Part model, mm, in its own coordinate system. Round coordinates to 2 decimals unless told otherwise and drop trailing zeros. Write each loop counter-clockwise with the first axis right and the second up, starting at its lowest first coordinate (ties: lowest second). Pieces come first, ordered by that corner, then holes. Notation, with made-up numbers: M 25,-24 L 48,-24 A9 ccw 48,-14 Z; hole C 15.25,46.5 d6. An arc over 180 degrees is marked long. Use one line per item in the form item = value. Start each with the question number.
Item 1: Flat gauge pins, fed straight in: pin 1 Ø3 at (y, z) = (3, 59) entering from +X; pin 2 Ø1.9 at (y, z) = (4.5, 45.5) entering from -X. Where does each tip first touch, or does it go through?
Item 2: Cut at A-A, the plane y = 4.5. State how many separate pieces and enclosed holes the cut face has, then the cut area to 3 significant figures.
Item 3: Probe L1, parallel to X at y = 2.5, z = 107; L2, parallel to X at y = 2.75, z = 9; L3, parallel to Z at x = 50.5, y = 3.25. List the from-to ranges inside material, lowest first.
Item 4: Cut at C-C, the plane x = 3. Give the cut face in (y, z), then the cut area to 3 significant figures.
Item 5: Cut at B-B, the plane z = 47. Give the cut face in (x, y).
Item 6: Cut at D-D, the plane z = 7. Give the cut face in (x, y).
from build123d import *

# Parameters (mm, degrees)
SKETCH1_R           = 2.6
SKETCH1_R_2         = 4
SKETCH1_R_3         = 6.35
SKETCH1_R_4         = 1
BOSS_EXTRUDE2_DEPTH = 6.3


with BuildPart() as part:
    # Sketch1 → Boss-Extrude2 (new body)
    with BuildSketch(Plane(origin=(0, 0, 0), x_dir=(1, 0, 0), z_dir=(0, 1, 0))):
        with BuildLine():
            Line((-65, 0), (65, 0))
            ThreePointArc((65, 0), (74, -9), (65, -18))
            Line((65, -18), (60, -18))
            ThreePointArc((60, -18), (57.878679656, -18.878679656), (57, -21))
            Line((57, -21), (57, -107))
            ThreePointArc((57, -107), (54.949747468, -111.949747468), (50, -114))
            Line((50, -114), (-50, -114))
            ThreePointArc((-50, -114), (-54.949747468, -111.949747468), (-57, -107))
            Line((-57, -107), (-57, -21))
            ThreePointArc((-57, -21), (-57.878679656, -18.878679656), (-60, -18))
            Line((-60, -18), (-65, -18))
            ThreePointArc((-65, -18), (-74, -9), (-65, 0))
        make_face()
        with Locations(Location((-50, -107, 0), (0, 0, 90))):
            Circle(SKETCH1_R, mode=Mode.SUBTRACT)
        with Locations(Location((50, -7, 0), (0, 0, 270))):
            Circle(SKETCH1_R, mode=Mode.SUBTRACT)
        with Locations(Location((65, -9, 0), (0, 0, 270))):
            Circle(SKETCH1_R_2, mode=Mode.SUBTRACT)
        with Locations(Location((50, -107, 0), (0, 0, 270))):
            Circle(SKETCH1_R, mode=Mode.SUBTRACT)
        with Locations(Location((0, -46.527767497, 0), (0, 0, 270))):
            Circle(SKETCH1_R_3, mode=Mode.SUBTRACT)
        with Locations(Location((0, -101.527767497, 0), (0, 0, 270))):
            Circle(SKETCH1_R_4, mode=Mode.SUBTRACT)
        with Locations(Location((-65, -9, 0), (0, 0, 90))):
            Circle(SKETCH1_R_2, mode=Mode.SUBTRACT)
        with Locations(Location((-50, -7, 0), (0, 0, 90))):
            Circle(SKETCH1_R, mode=Mode.SUBTRACT)
    extrude(amount=BOSS_EXTRUDE2_DEPTH)


solid = part.part
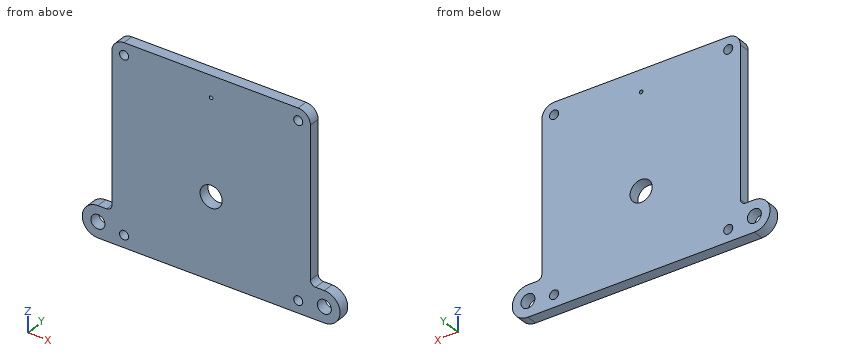
Model answer:
q1.pin_1 = 57
q1.pin_2 = -57
q2.separate_pieces = 1
q2.enclosed_holes = 8
q2.area = 13,200 mm²
q3.L1 = -57 to -52.6, -47.4 to 47.4, 52.6 to 57
q3.L2 = -74 to -69, -61 to -51.66, -48.34 to 48.34, 51.66 to 61, 69 to 74
q3.L3 = 0 to 4.45, 9.55 to 104.45, 109.55 to 113.98
q4.outline = M 0,0 L 6.3,0 L 6.3,40.93 L 0,40.93 Z; M 0,52.12 L 6.3,52.12 L 6.3,114 L 0,114 Z
q4.area = 648 mm²
q5.outline = M -57,0 L -6.33,0 L -6.33,6.3 L -57,6.3 Z; M 6.33,0 L 57,0 L 57,6.3 L 6.33,6.3 Z
q6.outline = M -73.77,0 L -68.46,0 L -68.46,6.3 L -73.77,6.3 Z; M -61.54,0 L -52.6,0 L -52.6,6.3 L -61.54,6.3 Z; M -47.4,0 L 47.4,0 L 47.4,6.3 L -47.4,6.3 Z; M 52.6,0 L 61.54,0 L 61.54,6.3 L 52.6,6.3 Z; M 68.46,0 L 73.77,0 L 73.77,6.3 L 68.46,6.3 Z
